```python
from build123d import *

# Parameters (mm, degrees)
F1_DEPTH  = 1.905
F3_DEPTH  = 3.811
F4_W      = 53.975
F4_H      = 107.315
F5_DEPTH  = 0.635
F6_W      = 15.875
F6_H      = 3.81
F7_DEPTH  = 3.811
F8_R      = 1.27
F9_R      = 4.7625
F10_DEPTH = 3.811


with BuildPart() as f1:
    # F0 (on Front) → F1 (new body, symmetric)
    with BuildSketch(Plane.XZ):
        with BuildLine():
            Line((-31.75, -57.15), (31.75, -57.15))
            ThreePointArc((31.75, -57.15), (36.240128, -55.290128), (38.1, -50.8))
            Line((38.1, -50.8), (38.1, 50.8))
            ThreePointArc((38.1, 50.8), (36.240128, 55.290128), (31.75, 57.15))
            Line((31.75, 57.15), (-31.75, 57.15))
            ThreePointArc((-31.75, 57.15), (-36.240128, 55.290128), (-38.1, 50.8))
            Line((-38.1, 50.8), (-38.1, -50.8))
            ThreePointArc((-38.1, -50.8), (-36.240128, -55.290128), (-31.75, -57.15))
        make_face()
    extrude(amount=F1_DEPTH, both=True)

    # F2 (on face) → F3 (cut, through all)
    with BuildSketch(Plane.XZ.offset(1.905)):
        with BuildLine():
            Line((19.05, 33.655), (-19.05, 33.655))
            ThreePointArc((-19.05, 33.655), (-23.540128, 31.795128), (-25.4, 27.305))
            Line((-25.4, 27.305), (-25.4, -41.275))
            ThreePointArc((-25.4, -41.275), (-23.540128, -45.765128), (-19.05, -47.625))
            Line((-19.05, -47.625), (19.05, -47.625))
            ThreePointArc((19.05, -47.625), (23.540128, -45.765128), (25.4, -41.275))
            Line((25.4, -41.275), (25.4, 27.305))
            ThreePointArc((25.4, 27.305), (23.540128, 31.795128), (19.05, 33.655))
        make_face()
    extrude(amount=-F3_DEPTH, mode=Mode.SUBTRACT)

    # F4 (on Front) → F5 (cut, symmetric)
    with BuildSketch(Plane.XZ):
        with Locations((0, 3.4925)):
            Rectangle(F4_W, F4_H)
    extrude(amount=F5_DEPTH, both=True, mode=Mode.SUBTRACT)

    # F6 (on face) → F7 (cut, through all)
    with BuildSketch(Plane.XZ.offset(1.905)):
        with Locations((0, 45.085)):
            Rectangle(F6_W, F6_H)
    extrude(amount=-F7_DEPTH, mode=Mode.SUBTRACT)

    # F8
    f8_edges = [f1.edges().sort_by_distance(p)[0] for p in [
        (-7.9375, 1.27, 46.99),
        (-7.9375, -1.27, 46.99),
        (7.9375, 1.27, 46.99),
        (7.9375, -1.27, 46.99),
        (7.9375, 1.27, 43.18),
        (7.9375, -1.27, 43.18),
        (-7.9375, 1.27, 43.18),
        (-7.9375, -1.27, 43.18),
    ]]
    fillet(f8_edges, radius=F8_R)

    # F9 (on face) → F10 (cut, through all)
    with BuildSketch(Plane.XZ.offset(1.905)):
        with Locations((-28.575, 47.625)):
            Circle(F9_R)
        with Locations((28.575, 47.625)):
            Circle(F9_R)
    extrude(amount=-F10_DEPTH, mode=Mode.SUBTRACT)


solid = f1.part
```
Design review of the part built by this model. Coordinates are the model's own, in mm. A direction names the side the tool comes from. Coordinates: 2 decimals unless noted, no trailing zeros. Order: outer loops, then holes, each group sorted by start corner. A loop starts at its lowest first (then second) coordinate and runs counter-clockwise, first axis right, second up.
1) Take a section at C-C, the plane x = 3.5. Give the boundary of the cut face in (y, z) (3 decimals).
2) Wall thickness on line 1 along Z through (x, y) = (14.5, 1.15) (3 decimals); line 2 along X through (y, z) = (1.05, -33); line 3 along X through (y, z) = (0.55, 28): over which ranges is each line inside the solid? List them lowest first.
3) For faces 4 (the flat face through (0, -0.635, 36)), 5 (the cylindrical face through (23.589, 1.261, 31.745)), 6 (the cylindrical face through (-36.19, -0.03, 55.34)), list the 3-axis set-ups (+Z, -Z, +X, -X, +Y, -Y) from which the entire face can be reached by the end or side of a thin tool; tool diameter is ignored.
4) Mouldability with a two-part tool opening along X and no side actions: class faces 1 (the cylindrical face through (36.29, -0.03, 55.24)), 2 (the cylindrical face through (-23.49, -1.279, 31.844)), 3 (the flat face through (0, 0, -57.15)) as +X half, -X half, draft (parallel to the pull), parting line (faces both ways), or undercut.
5) Take a section at B-B, the plane z = -6.5. Give the boundary of the cut face in (x, y) (1 decimal), and give its area (3 significant figures).
6) Take a section at A-A, the plane x = -17.5. Give the boundary of the cut face in (y, z) (3 decimals).
7) Take a section at D-D, the plane x = 21. Give the boundary of the cut face in (y, z) (3 decimals), and give its area (3 significant figures).
8) Clearance check with flat-ended pins moving along their axes: pin 1 (6 mm diameter, centred on x = -24, z = 18.5, fed in from +Y) (3 decimals); pin 2 (10 mm diameter, centred on x = -19.5, z = -27, fed in from -Y). State where each tip first meets the part, or that it passes through.
Returned:
1. outline: (-1.905, -57.15) - (1.905, -57.15) - (1.905, -47.625) - (0.635, -47.625) - (0.635, -50.165) - (-0.635, -50.165) - (-0.635, -47.625) - (-1.905, -47.625) - close; (-1.905, 33.655) - (-0.635, 33.655) - (-0.635, 43.18) - (-1.905, 43.18) - close; (-1.905, 46.99) - (-0.635, 46.99) - (-0.635, 57.15) - (-1.905, 57.15) - close; (0.635, 33.655) - (1.905, 33.655) - (1.905, 43.18) - (0.635, 43.18) - close; (0.635, 46.99) - (1.905, 46.99) - (1.905, 57.15) - (0.635, 57.15) - close
2. line 1: z = -57.15 to -47.625, 33.655 to 57.15
2. line 2: x = -38.1 to -25.4, 25.4 to 38.1
2. line 3: x = -38.1 to -26.99, 26.99 to 38.1
3. face 4: +Z
3. face 5: +Y, -Y
3. face 6: +Z, -X, +Y, -Y
4. face 1: +X half
4. face 2: undercut
4. face 3: draft
5. outline: (-38.1, -1.9) - (-25.4, -1.9) - (-25.4, -0.6) - (-27, -0.6) - (-27, 0.6) - (-25.4, 0.6) - (-25.4, 1.9) - (-38.1, 1.9) - close; (25.4, -1.9) - (38.1, -1.9) - (38.1, 1.9) - (25.4, 1.9) - (25.4, 0.6) - (27, 0.6) - (27, -0.6) - (25.4, -0.6) - close
5. area: 92.7 mm2
6. outline: (-1.905, -57.15) - (1.905, -57.15) - (1.905, -47.625) - (0.635, -47.625) - (0.635, -50.165) - (-0.635, -50.165) - (-0.635, -47.625) - (-1.905, -47.625) - close; (-1.905, 33.655) - (-0.635, 33.655) - (-0.635, 57.15) - (-1.905, 57.15) - close; (0.635, 33.655) - (1.905, 33.655) - (1.905, 57.15) - (0.635, 57.15) - close
7. outline: (-1.905, -57.15) - (1.905, -57.15) - (1.905, -47.318) - (0.635, -47.318) - (0.635, -50.165) - (-0.635, -50.165) - (-0.635, -47.318) - (-1.905, -47.318) - close; (-1.905, 33.348) - (-0.635, 33.348) - (-0.635, 57.15) - (-1.905, 57.15) - close; (0.635, 33.348) - (1.905, 33.348) - (1.905, 57.15) - (0.635, 57.15) - close
7. area: 94.3 mm2
8. pin 1: stops at y = 1.905
8. pin 2: passes through
